Part print with two shaded views. Sizes in mm from the minimum x, y, z corner. A direction names the side the tool comes from. Give positions to 0.01 mm unless a question says otherwise; leave off trailing zeros. Write each loop counter-clockwise with the first axis right and the second up, starting at its lowest first coordinate (ties: lowest second). Pieces come first, ordered by that corner, then holes.
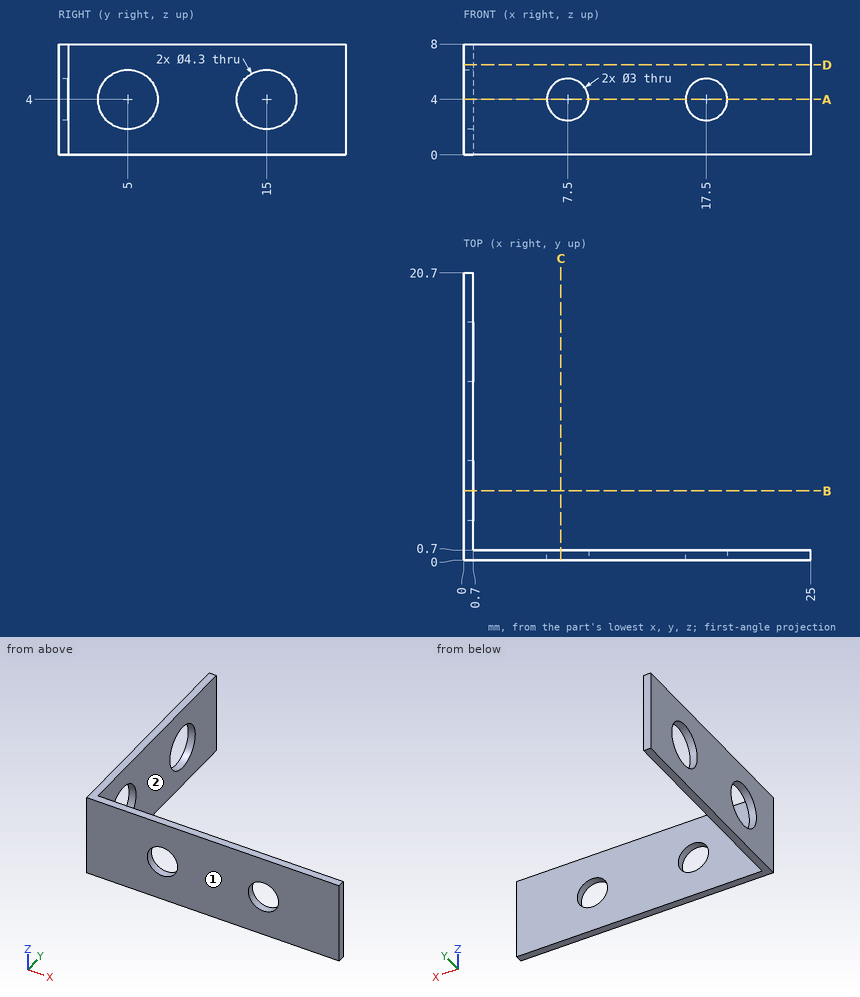
1) Pin check, flat tips, straight feed: pin 1 Ø1.8 at (x, z) = (17.5, 4) entering from -Y; pin 2 Ø1.5 at (x, z) = (20, 6.5) entering from +Y; pin 3 Ø3 at (y, z) = (11.5, 4.5) entering from +X. Stop position of each tip, or through.
Answers follow:
pin 1: passes through
pin 2: stops at y = 0.7
pin 3: stops at x = 0.7
2) Saw through at A-A, the plane z = 4. Write the cut outline in (x, y), then the cut area to 3 significant figures.
Answers follow:
outline: (0, 0) - (6, 0) - (6, 0.7) - (0.7, 0.7) - (0.7, 2.85) - (0, 2.85) - close; (0, 7.15) - (0.7, 7.15) - (0.7, 12.85) - (0, 12.85) - close; (0, 17.15) - (0.7, 17.15) - (0.7, 20.7) - (0, 20.7) - close; (9, 0) - (16, 0) - (16, 0.7) - (9, 0.7) - close; (19, 0) - (25, 0) - (25, 0.7) - (19, 0.7) - close
area: 21.3 mm2
3) 3-axis set-ups, long thin cutter, end or side, ignore diameter. For the marked faces 1 and 2: which of +Z, -Z, +X, -X, +Y, -Y reach the whole face in a straight line?
Answers follow:
face 1: +Z, -Z, +X, -X, -Y
face 2: +Z, -Z, +X, +Y
4) Saw through at B-B, the plane y = 5. Write the cut outline in (x, z).
Answers follow:
outline: (0, 0) - (0.7, 0) - (0.7, 1.85) - (0, 1.85) - close; (0, 6.15) - (0.7, 6.15) - (0.7, 8) - (0, 8) - close
5) Saw through at D-D, the plane z = 6.5. Write the cut outline in (x, y), then the cut area to 3 significant figures.
Answers follow:
outline: (0, 0) - (25, 0) - (25, 0.7) - (0.7, 0.7) - (0.7, 20.7) - (0, 20.7) - close
area: 31.5 mm2
6) Wall check: L1, parallel to Y at x = 0.25, z = 4; L2, parallel to Z at x = 7.5, y = 0.4; L3, parallel to X at y = 0.2, z = 4. Give the ranges that are in metal, low to high.
Answers follow:
L1: y = 0 to 2.85, 7.15 to 12.85, 17.15 to 20.7
L2: z = 0 to 2.5, 5.5 to 8
L3: x = 0 to 6, 9 to 16, 19 to 25
7) Saw through at C-C, the plane x = 7. Write the cut outline in (y, z), then the cut area to 3 significant figures.
Answers follow:
outline: (0, 0) - (0.7, 0) - (0.7, 2.59) - (0, 2.59) - close; (0, 5.41) - (0.7, 5.41) - (0.7, 8) - (0, 8) - close
area: 3.62 mm2
